```python
from build123d import *

# Parameters (mm, degrees)
SKETCH_1_W      = 27.9
SKETCH_1_H      = 55.5
SKETCH_1_R      = 1.5
EXTRUDE_1_DEPTH = 1.6
SKETCH_2_W      = 6.9
SKETCH_2_H      = 6.9
SKETCH_2_W_2    = 6.4
SKETCH_2_H_2    = 3.5
EXTRUDE_2_DEPTH = 1.6
EXTRUDE_3_DEPTH = 3.5
SKETCH_4_W      = 2
SKETCH_4_H      = 1
SKETCH_4_W_2    = 1
SKETCH_4_H_2    = 2
EXTRUDE_4_DEPTH = 0.5


with BuildPart() as part:
    # Эскиз1 → Бобышка-Вытянуть1 (new body)
    with BuildSketch(Plane(origin=(0, 0, 0), x_dir=(1, 0, 0), z_dir=(0, 1, 0))):
        Rectangle(SKETCH_1_W, SKETCH_1_H)
        with Locations(Location((-11.45, 25.15, 0), (0, 0, 270))):
            Circle(SKETCH_1_R, mode=Mode.SUBTRACT)
        with Locations(Location((11.45, 25.15, 0), (0, 0, 270))):
            Circle(SKETCH_1_R, mode=Mode.SUBTRACT)
    extrude(amount=EXTRUDE_1_DEPTH)

    # Эскиз2 → Бобышка-Вытянуть2 (add)
    with BuildSketch(Plane(origin=(0, 1.6, 0), x_dir=(1, 0, 0), z_dir=(0, 1, 0))):
        with Locations((-2.1, -3.8)):
            Rectangle(SKETCH_2_W, SKETCH_2_H)
        with Locations((-7.15, -21)):
            Rectangle(SKETCH_2_W_2, SKETCH_2_H_2)
    extrude(amount=EXTRUDE_2_DEPTH)

    # Эскиз3 → Бобышка-Вытянуть3 (add)
    with BuildSketch(Plane(origin=(0, 1.6, 0), x_dir=(1, 0, 0), z_dir=(0, 1, 0))):
        with BuildLine():
            Line((2.55, -14.35), (-3.85, -14.35))
            ThreePointArc((-3.85, -14.35), (-5.65, -12.55), (-3.85, -10.75))
            Line((-3.85, -10.75), (2.55, -10.75))
            ThreePointArc((2.55, -10.75), (4.35, -12.55), (2.55, -14.35))
        make_face()
    extrude(amount=EXTRUDE_3_DEPTH)

    # Эскиз4 → Бобышка-Вытянуть4 (add)
    with BuildSketch(Plane(origin=(0, 1.6, 0), x_dir=(1, 0, 0), z_dir=(0, 1, 0))):
        with Locations((10.25, -20.95)):
            Rectangle(SKETCH_4_W, SKETCH_4_H)
        with Locations((10.25, -18.721428571)):
            Rectangle(SKETCH_4_W, SKETCH_4_H)
        with Locations((10.25, -16.492857143)):
            Rectangle(SKETCH_4_W, SKETCH_4_H)
        with Locations((10.25, -14.264285714)):
            Rectangle(SKETCH_4_W, SKETCH_4_H)
        with Locations((10.25, -12.035714286)):
            Rectangle(SKETCH_4_W, SKETCH_4_H)
        with Locations((10.25, -9.807142857)):
            Rectangle(SKETCH_4_W, SKETCH_4_H)
        with Locations((10.25, -7.578571429)):
            Rectangle(SKETCH_4_W, SKETCH_4_H)
        with Locations((10.25, -5.35)):
            Rectangle(SKETCH_4_W, SKETCH_4_H)
        with Locations((10.25, -3.121428571)):
            Rectangle(SKETCH_4_W, SKETCH_4_H)
        with Locations((10.25, -0.892857143)):
            Rectangle(SKETCH_4_W, SKETCH_4_H)
        with Locations((10.25, 1.335714286)):
            Rectangle(SKETCH_4_W, SKETCH_4_H)
        with Locations((10.25, 3.564285714)):
            Rectangle(SKETCH_4_W, SKETCH_4_H)
        with Locations((10.25, 5.792857143)):
            Rectangle(SKETCH_4_W, SKETCH_4_H)
        with Locations((10.25, 8.021428571)):
            Rectangle(SKETCH_4_W, SKETCH_4_H)
        with Locations((10.25, 10.25)):
            Rectangle(SKETCH_4_W, SKETCH_4_H)
        with Locations((-10.25, 7.25)):
            Rectangle(SKETCH_4_W_2, SKETCH_4_H_2)
        with Locations((-8.472222222, 7.25)):
            Rectangle(SKETCH_4_W_2, SKETCH_4_H_2)
        with Locations((-6.694444444, 7.25)):
            Rectangle(SKETCH_4_W_2, SKETCH_4_H_2)
        with Locations((-4.916666667, 7.25)):
            Rectangle(SKETCH_4_W_2, SKETCH_4_H_2)
        with Locations((-3.138888889, 7.25)):
            Rectangle(SKETCH_4_W_2, SKETCH_4_H_2)
        with Locations((-1.361111111, 7.25)):
            Rectangle(SKETCH_4_W_2, SKETCH_4_H_2)
        with Locations((0.416666667, 7.25)):
            Rectangle(SKETCH_4_W_2, SKETCH_4_H_2)
        with Locations((2.194444444, 7.25)):
            Rectangle(SKETCH_4_W_2, SKETCH_4_H_2)
        with Locations((3.972222222, 7.25)):
            Rectangle(SKETCH_4_W_2, SKETCH_4_H_2)
        with Locations((5.75, 7.25)):
            Rectangle(SKETCH_4_W_2, SKETCH_4_H_2)
        with Locations((5.35, 3.35)):
            Rectangle(SKETCH_4_W, SKETCH_4_H)
        with Locations((5.35, 1.6)):
            Rectangle(SKETCH_4_W, SKETCH_4_H)
        with Locations((5.35, -0.15)):
            Rectangle(SKETCH_4_W, SKETCH_4_H)
        with Locations((-10.25, 0.75)):
            Rectangle(SKETCH_4_W, SKETCH_4_H)
        with Locations((-10.25, 3.05)):
            Rectangle(SKETCH_4_W, SKETCH_4_H)
        with Locations((-10.25, -1.55)):
            Rectangle(SKETCH_4_W, SKETCH_4_H)
        with Locations((-10.25, -3.85)):
            Rectangle(SKETCH_4_W, SKETCH_4_H)
        with Locations((-10.25, -6.15)):
            Rectangle(SKETCH_4_W, SKETCH_4_H)
    extrude(amount=EXTRUDE_4_DEPTH)


solid = part.part
```
Verification items for the finished model (mm, model axes). A direction names the side the tool comes from. Round coordinates to 2 decimals unless told otherwise and drop trailing zeros. Order: outer loops, then holes, each group sorted by start corner. A loop starts at its lowest first (then second) coordinate and runs counter-clockwise, first axis right, second up. Notation, with made-up numbers: (-2.75, 44.5) -> (56.25, 44.5) arc R15 ccw to (56.25, 61.5) -> close; hole circle Ø3 at (26.25, 5.25). An arc over 180 degrees is marked (long way). Put each result on its own line as item: value. Start each with the question number.
(1) Material ranges on line 1 along X through (y, z) = (0.8, -25.15); line 2 along Y through (x, z) = (4.5, -12.5); line 3 along Y through (x, z) = (-8.75, 19.5), recorded low to high.
(2) Tool access check on faces 1 (the face through (10, 2.1, 21)), 2 (the face through (-10.35, 2, 21)), 3 (the face through (-10, 2.1, 4)), 4 (the face through (-7, 3.2, 21)). Record the directions out of +Z, -Z, +X, -X, +Y, -Y that give a thin tool (end or side, any length) a straight path to the whole face; none if there is none.
(3) Draft check along Z on faces 5 (the face through (0, 1, -27.75)), 6 (the face through (-5, 2.1, -7)), 7 (the face through (-11.38, 0.79, -26.65)). Enter one of: +Z half, -Z half, draft (parallel to the pull), parting line (faces both ways), or undercut.
(4) Depth check by flat-ended pin: pin 1 Ø1.1 at (x, z) = (10, 19) entering from +Y; pin 2 Ø3 at (y, z) = (4, 19.5) entering from +X; pin 3 Ø0.6 at (x, y) = (10.5, 2) entering from +Z. Enter the tip coordinate at first touch or a pass-through.
(5) Section check B-B (z = -25.15). Enter the section's corners in (x, y), then the cut area to 3 significant figures.
(6) Section check C-C (z = -15). Enter the section's corners in (x, y), then the cut area to 3 significant figures.
(7) Section check A-A (y = 2.6). Enter the section's corners in (x, z).
Completed:
1. line 1: x = -13.95 to -12.95, -9.95 to 9.95, 12.95 to 13.95
1. line 2: y = 0 to 1.6
1. line 3: y = 0 to 3.2
2. face 1: +Z, -Z, +X, +Y
2. face 2: +Z, -X, +Y
2. face 3: -Z, -X, +Y
2. face 4: +Z, +X, -X, +Y
3. face 5: -Z half
3. face 6: draft
3. face 7: undercut
4. pin 1: stops at y = 2.1
4. pin 2: stops at x = -3.95
4. pin 3: stops at z = 21.45
5. outline: (-13.95, 0) -> (-12.95, 0) -> (-12.95, 1.6) -> (-13.95, 1.6) -> close; (-9.95, 0) -> (9.95, 0) -> (9.95, 1.6) -> (-9.95, 1.6) -> close; (12.95, 0) -> (13.95, 0) -> (13.95, 1.6) -> (12.95, 1.6) -> close
5. area: 35.0 mm2
6. outline: (-13.95, 0) -> (13.95, 0) -> (13.95, 1.6) -> (-13.95, 1.6) -> close
6. area: 44.6 mm2
7. outline: (-10.35, 19.25) -> (-3.95, 19.25) -> (-3.95, 22.75) -> (-10.35, 22.75) -> close; (-5.55, 0.35) -> (1.35, 0.35) -> (1.35, 7.25) -> (-5.55, 7.25) -> close; (-3.85, 10.75) -> (2.55, 10.75) arc R1.8 ccw to (2.55, 14.35) -> (-3.85, 14.35) arc R1.8 ccw to start
